Verification items for the finished model (mm, model axes). A direction names the side the tool comes from. Coordinates: 2 decimals unless noted, no trailing zeros. Write each loop counter-clockwise with the first axis right and the second up, starting at its lowest first coordinate (ties: lowest second). Pieces come first, ordered by that corner, then holes. Notation, with made-up numbers: (51, -36.75) - (90, -36.75) arc R17 ccw to (90, -21.75) - close; hole circle Ø1 at (83.25, 63). An arc over 180 degrees is marked (long way). Answer as CSV lines item,"result". Start each with the question number.
Autodesk Inventor part; units mm, degrees
ref_plane "YZ Plane" through (0, 0, 0) normal (1, 0, 0) x (0, 1, 0)
ref_plane "XZ Plane" through (0, 0, 0) normal (0, 1, 0) x (-1, 0, 0)
ref_plane "XY Plane" through (0, 0, 0) normal (0, 0, 1) x (1, 0, 0)
sketch "Sketch1" plane through (0, 0, 0) normal (0, 1, 0) x (-1, 0, 0)
  line L0 (0, -8) -> (15, -8)
  line L1 (15, -8) -> (15, 0)
  line L2 (15, 0) -> (0, 0)
  line L3 (0, 0) -> (0, -8)
  line L4 (7.5, 0) -> (7.5, -8) construction
  line L5 (0, -4) -> (15, -4) construction
  line L6 (3.5, 0) -> (3.5, -8)
  line L7 (11.5, -8) -> (11.5, 0)
  circle A0 centre (7.5, -4) radius 2.4
  circle A1 centre (7.5, -4) radius 4
  dimension "d2" = 15
  dimension "d3" = 8
  dimension "d4" = 4
  dimension "d5" = 4
  dimension "d6" = 4.8
  dimension "d7" = 8
extrude "Extrusion1" add sketch "Sketch1" along normal blind 4 contours L3 L2 L6 L0 | L7 L2 L1 L0
extrude "Extrusion2" add sketch "Sketch1" along normal blind 7.8 contours L6 A1 L0 | A1 L7 L0 | A1 | L6 L2 A1 | A1 L2 L7
extrude "Extrusion3" add sketch "Sketch1" along normal blind 10.1 from surface at 7.8 contours A1
equation "\"d4\" = 0.5 * d3"
equation "\"d5\" = 0.5 * d3"
properties part number "diff_gear_holder_3"
1. Draft check along X on faces 6 (the face through (0, 2, -4)), 7 (the face through (-8.79, 8.825, -6.024)), 8 (the face through (-11.5, 6, -4)). Enter one of: pulls with the +X half, pulls with the -X half, needs draft (parallel to the pull), parting line crosses it, or undercut.
2. Cross-section at A-A (z = -6). Record the cut outline in (x, y).
3. Cross-section at C-C (z = -0.5). Record the cut outline in (x, y).
4. Depth check by flat-ended pin: P1, Ø1, axis at y = 12, z = -6, coming from the +X side; P2, Ø1.5, axis at y = 15.5, z = -1, coming from the -X side; P3, Ø1.1, axis at y = 6, z = -4, coming from the +X side; P4, Ø4, axis at x = -7.5, z = -4, coming from the -Y side. Enter the tip coordinate at first touch or a pass-through.
5. Cross-section at B-B (y = 3.5). Record the cut outline in (x, z).
6. Access from +Z, -Z, +X, -X, +Y, -Y to the whole of each face (thin tool, end or side, straight path). Record for faces 1 (the face through (-13, 4, -4)), 2 (the face through (-11, 7.8, -1)), 3 (the face through (-11, 7.8, -7)), 4 (the face through (-2, 4, -4)), 5 (the face through (-6.633, 12.779, -0.095)).
7. Scan lines: line 1 along Z through (x, y) = (-7.5, 6); line 2 along Y through (x, z) = (-4, -2); line 3 along Y through (x, z) = (-1.5, -2.75). Record each from-to range of solid material in increasing order. Write a range as from..to.
Completed:
1,face 6,"pulls with the +X half"
1,face 7,"undercut"
1,face 8,"pulls with the -X half"
2,outline,"(-15, 0) - (-8.83, 0) - (-8.83, 17.9) - (-10.96, 17.9) - (-10.96, 7.8) - (-11.5, 7.8) - (-11.5, 4) - (-15, 4) - close; (-6.17, 0) - (0, 0) - (0, 4) - (-3.5, 4) - (-3.5, 7.8) - (-4.04, 7.8) - (-4.04, 17.9) - (-6.17, 17.9) - close"
3,outline,"(-15, 0) - (0, 0) - (0, 4) - (-3.5, 4) - (-3.5, 7.8) - (-5.56, 7.8) - (-5.56, 17.9) - (-9.44, 17.9) - (-9.44, 7.8) - (-11.5, 7.8) - (-11.5, 4) - (-15, 4) - close"
4,P1,"stops at x = -3.79"
4,P2,"stops at x = -10.81"
4,P3,"stops at x = -3.5"
4,P4,"passes through"
5,outline,"(-15, -8) - (0, -8) - (0, 0) - (-15, 0) - close; hole circle Ø4.8 at (-7.5, -4)"
6,face 1,"+Z, -Z, -X, +Y"
6,face 2,"+Z, -X, +Y"
6,face 3,"-Z, -X, +Y"
6,face 4,"+Z, -Z, +X, +Y"
6,face 5,"+Y"
7,line 1,"z = -8..-6.4, -1.6..0"
7,line 2,"y = 0..7.8"
7,line 3,"y = 0..4"
